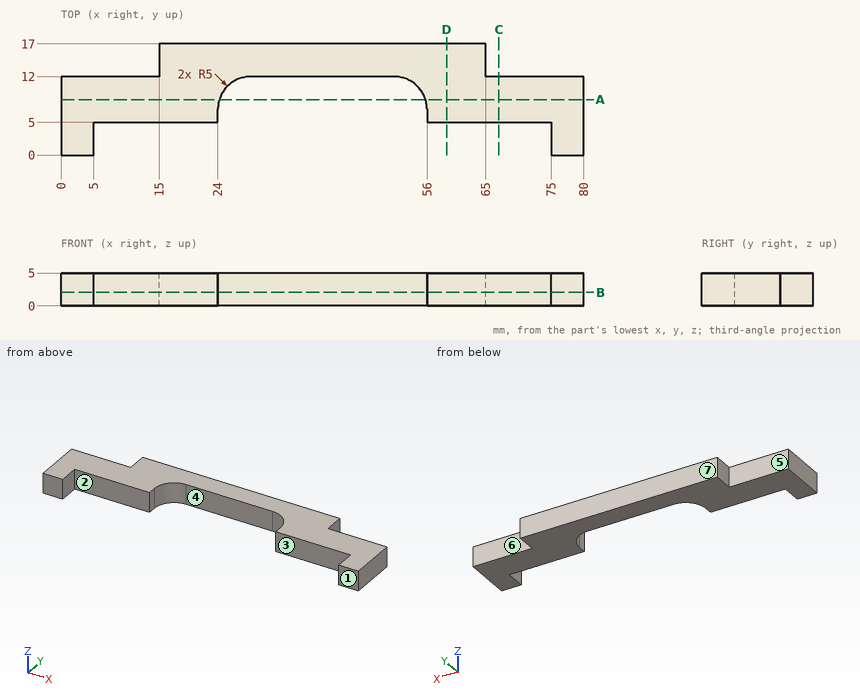
Geometry check sheet. Reference: drawing and pictorial views, mm from the part's lowest x, y, z. A direction names the side the tool comes from. Round coordinates to 2 decimals unless told otherwise and drop trailing zeros. Write each loop counter-clockwise with the first axis right and the second up, starting at its lowest first coordinate (ties: lowest second). Pieces come first, ordered by that corner, then holes.
1. Section check B-B on z = 2.05. Enter the section's corners in (x, y), plus the area to 3 significant figures.
2. Draft check along X on the marked faces 1, 2 and 3. Enter one of: +X half, -X half, draft (parallel to the pull), parting line (faces both ways), or undercut.
3. Gauge pin test, flat ends, axial feed: P1, Ø1.6, axis at y = 5.5, z = 3.5, coming from the -X side; P2, Ø2.5, axis at x = 74.5, z = 2, coming from the +Y side; P3, Ø1.5, axis at y = 13.5, z = 2, coming from the +X side; P4, Ø1.5, axis at y = 15, z = 3.5, coming from the -X side. Record the tip position at first contact, or that the pin passes through.
4. Section check D-D on x = 59. Enter the section's corners in (y, z).
5. Section check C-C on x = 67. Enter the section's corners in (y, z), plus the area to 3 significant figures.
6. Access from +Z, -Z, +X, -X, +Y, -Y to the whole of each face (thin tool, end or side, straight path). Record for the marked faces 4, 5, 6 and 7.
7. Section check A-A on y = 8.5. Enter the section's corners in (x, z), plus the area to 3 significant figures.
8. Scan lines: L1, parallel to X at y = 4.5, z = 4.3; L2, parallel to X at y = 6.75, z = 3.1; L3, parallel to X at y = 12.5, z = 2.9. Record each from-to range of solid material in increasing order.
Answer:
1. outline: (0, 0) - (5, 0) - (5, 5) - (24, 5) - (24, 7) arc R5 cw to (29, 12) - (51, 12) arc R5 cw to (56, 7) - (56, 5) - (75, 5) - (75, 0) - (80, 0) - (80, 12) - (65, 12) - (65, 17) - (15, 17) - (15, 12) - (0, 12) - close
1. area: 647 mm2
2. face 1: draft
2. face 2: undercut
2. face 3: undercut
3. P1: stops at x = 0
3. P2: stops at y = 12
3. P3: stops at x = 65
3. P4: stops at x = 15
4. outline: (5, 0) - (17, 0) - (17, 5) - (5, 5) - close
5. outline: (5, 0) - (12, 0) - (12, 5) - (5, 5) - close
5. area: 35.0 mm2
6. face 4: +Z, -Z, -Y
6. face 5: +Z, -Z, -X, +Y
6. face 6: +Z, -Z, +X, +Y
6. face 7: +Z, -Z, +X, -X, +Y
7. outline: (0, 0) - (24.23, 0) - (24.23, 5) - (0, 5) - close; (55.77, 0) - (80, 0) - (80, 5) - (55.77, 5) - close
7. area: 242 mm2
8. L1: x = 0 to 5, 75 to 80
8. L2: x = 0 to 24, 56 to 80
8. L3: x = 15 to 65
